Geometry check sheet. Reference: the model listing, model coordinates, mm. A direction names the side the tool comes from. Coordinates: 2 decimals unless noted, no trailing zeros. Loops run counter-clockwise (first coordinate to the right, second up) from the corner with the lowest first, then second, coordinate; pieces in that order, holes last. Notation, with made-up numbers: M 84.5,71 L 98.5,71 A23 cw 98.5,101 Z; hole C 23.25,23.5 d5. An arc over 180 degrees is marked long. Use CSV: the item, a comma, the result in double quotes.
```python
from build123d import *

# Parameters (mm, degrees)
EXTRUDE_1_DEPTH     = 1
CUT_EXTRUDE_2_DEPTH = 0.5


with BuildPart() as part:
    # 草图1 → 凸台-拉伸1 (new body)
    with BuildSketch(Plane.XY):
        with BuildLine():
            Line((2, 0), (28.9, 0))
            ThreePointArc((28.9, 0), (30.314213562, 0.585786438), (30.9, 2))
            Line((30.9, 2), (30.9, 11.4))
            ThreePointArc((30.9, 11.4), (30.314213562, 12.814213562), (28.9, 13.4))
            Line((28.9, 13.4), (2, 13.4))
            ThreePointArc((2, 13.4), (0.585786438, 12.814213562), (0, 11.4))
            Line((0, 11.4), (0, 2))
            ThreePointArc((0, 2), (0.585786438, 0.585786438), (2, 0))
        make_face()
    extrude(amount=EXTRUDE_1_DEPTH)

    # 草图3 → 切除-拉伸2 (cut)
    with BuildSketch(Plane(origin=(0, 0, 0), x_dir=(-1, 0, 0), z_dir=(0, 0, -1))):
        with BuildLine():
            Line((-30.9, 13.4), (-27.9, 13.4))
            Line((-27.9, 13.4), (-27.9, 10.9))
            ThreePointArc((-27.9, 10.9), (-28.046446609, 10.546446609), (-28.4, 10.4))
            Line((-28.4, 10.4), (-30.9, 10.4))
            Line((-30.9, 10.4), (-30.9, 13.4))
        make_face()
        with BuildLine():
            Line((-3, 13.4), (-3, 10.9))
            ThreePointArc((-3, 10.9), (-2.853553391, 10.546446609), (-2.5, 10.4))
            Line((-2.5, 10.4), (0, 10.4))
            Line((0, 10.4), (0, 13.4))
            Line((0, 13.4), (-3, 13.4))
        make_face()
        with BuildLine():
            Line((0, 0), (-3, 0))
            Line((-3, 0), (-3, 2.5))
            ThreePointArc((-3, 2.5), (-2.853553391, 2.853553391), (-2.5, 3))
            Line((-2.5, 3), (0, 3))
            Line((0, 3), (0, 0))
        make_face()
        with BuildLine():
            Line((-27.9, 0), (-27.9, 2.5))
            ThreePointArc((-27.9, 2.5), (-28.046446609, 2.853553391), (-28.4, 3))
            Line((-28.4, 3), (-30.9, 3))
            Line((-30.9, 3), (-30.9, 0))
            Line((-30.9, 0), (-27.9, 0))
        make_face()
    extrude(amount=-CUT_EXTRUDE_2_DEPTH, mode=Mode.SUBTRACT)


solid = part.part
```
1. Section check A-A, the plane z = 0.35. Record the cut outline in (x, y), plus the area to 3 significant figures.
The answers:
outline,"M 0,3 L 2.5,3 A0.5 cw 3,2.5 L 3,0 L 27.9,0 L 27.9,2.5 A0.5 cw 28.4,3 L 30.9,3 L 30.9,10.4 L 28.4,10.4 A0.5 cw 27.9,10.9 L 27.9,13.4 L 3,13.4 L 3,10.9 A0.5 cw 2.5,10.4 L 0,10.4 Z"
area,"378 mm^2"
2. Section check C-C, the plane y = 1.5. Record the cut outline in (x, z), plus the area to 3 significant figures.
The answers:
outline,"M 0.06,0.5 L 3,0.5 L 3,0 L 27.9,0 L 27.9,0.5 L 30.84,0.5 L 30.84,1 L 0.06,1 Z"
area,"27.8 mm^2"
3. Gauge pin test, flat ends, axial feed: P1, Ø2.5, axis at x = 1, y = 12, coming from the -Z side; P2, Ø0.6, axis at x = 30, z = 0, coming from the -Y side; P3, Ø0.6, axis at y = 1, z = 0, coming from the -X side. Record the tip position at first contact, or that the pin passes through.
The answers:
P1,"z = 0.5"
P2,"y = 3"
P3,"x = 3"
4. Set-up check for faces 1 (the flat face through (2, 12, 0.5)), 2 (the flat face through (29, 12, 0.5)), 3 (the flat face through (1, 2, 0.5)), 4 (the flat face through (29, 2, 0.5)): record each of +Z, -Z, +X, -X, +Y, -Y from which the full face is reachable in a straight line by a thin tool's end or side.
The answers:
face 1,"-Z, -X, +Y"
face 2,"-Z, +X, +Y"
face 3,"-Z, -X, -Y"
face 4,"-Z, +X, -Y"
5. Section check B-B, the plane y = 12. Record the cut outline in (x, z).
The answers:
outline,"M 0.09,0.5 L 3,0.5 L 3,0 L 27.9,0 L 27.9,0.5 L 30.81,0.5 L 30.81,1 L 0.09,1 Z"
6. Thickness scan on line 1 (Z direction, x = 29, y = 12.5); line 2 (Y direction, x = 2.5, z = 0.2); line 3 (X direction, y = 12.25, z = 0.2). Record the ranges inside material, lowest first. Write a range as [from, to].
The answers:
line 1,"[0.5, 1]"
line 2,"[3, 10.4]"
line 3,"[3, 27.9]"
